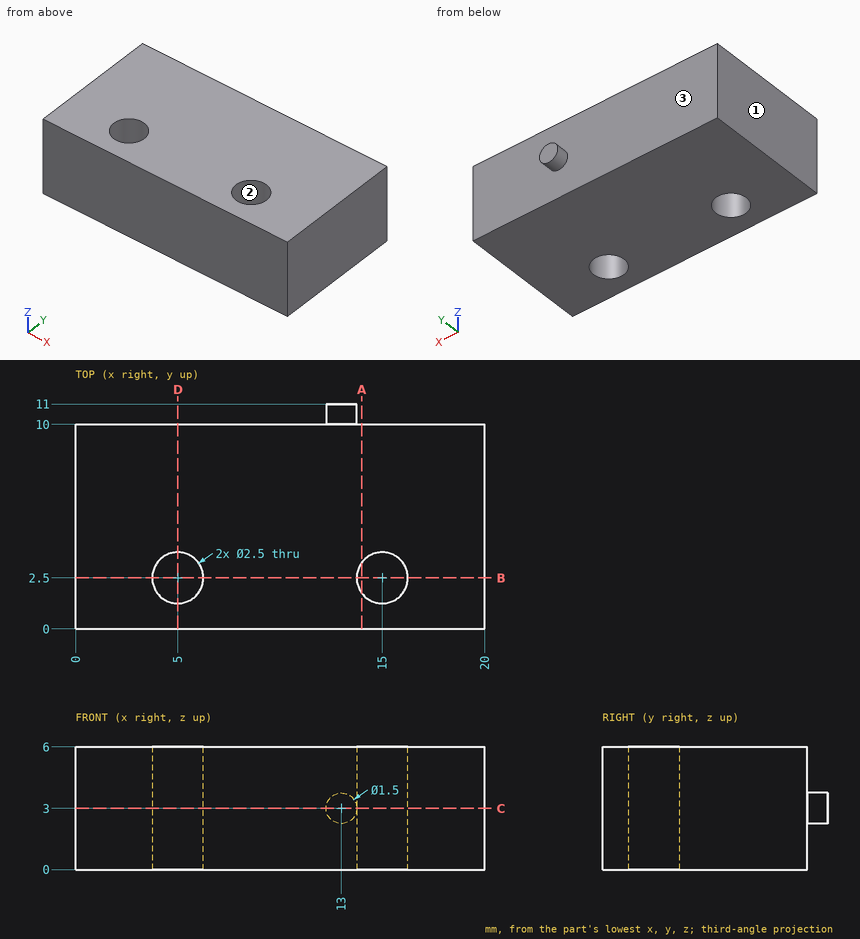
Could you check a few things on this drawing? It's one solid part, dimensions in mm from its lowest x, y, z. Give positions to 0.01 mm unless a question says otherwise; leave off trailing zeros. Write each loop counter-clockwise with the first axis right and the second up, starting at its lowest first coordinate (ties: lowest second). Pieces come first, ordered by that corner, then holes.
(1) Imagine slicing it at C-C, the plane z = 3. Write out the boundary of the cut face in (x, y).
Output values:
outline: (0, 0) - (20, 0) - (20, 10) - (13.75, 10) - (13.75, 11) - (12.25, 11) - (12.25, 10) - (0, 10) - close; hole circle Ø2.5 at (5, 2.5); hole circle Ø2.5 at (15, 2.5)
(2) If I drill on L1, parallel to Y at x = 5, z = 3.4; L2, parallel to X at y = 3.5, z = 4.35; L3, parallel to Y at x = 10.5, z = 1.85, over which ranges is the centre line in solid material (lowest first)?
Output values:
L1: y = 0 to 1.25, 3.75 to 10
L2: x = 0 to 4.25, 5.75 to 14.25, 15.75 to 20
L3: y = 0 to 10
(3) Imagine slicing it at A-A, the plane x = 14. Write out the boundary of the cut face in (y, z), and give its area (3 significant figures).
Output values:
outline: (0, 0) - (1.75, 0) - (1.75, 6) - (0, 6) - close; (3.25, 0) - (10, 0) - (10, 6) - (3.25, 6) - close
area: 51.0 mm2
(4) Will these pins go through, and if not, where does the flat tip stop? pin 1 (2 mm diameter, centred on x = 5, y = 2.5, fed in from -Z); pin 2 (2 mm diameter, centred on x = 15.5, y = 2, fed in from -Z); pin 3 (3 mm diameter, centred on x = 9, z = 4, fed in from +Y).
Output values:
pin 1: passes through
pin 2: stops at z = 0
pin 3: stops at y = 10
(5) Thinking about a two-plate mould opening in Y: for the marked faces 1, 2 and 3, which applies, pulls with the +Y half, pulls with the -Y half, needs draft (parallel to the pull), parting line crosses it, or undercut?
Output values:
face 1: needs draft
face 2: undercut
face 3: pulls with the +Y half
(6) Imagine slicing it at D-D, the plane x = 5. Write out the boundary of the cut face in (y, z), and give its area (3 significant figures).
Output values:
outline: (0, 0) - (1.25, 0) - (1.25, 6) - (0, 6) - close; (3.75, 0) - (10, 0) - (10, 6) - (3.75, 6) - close
area: 45.0 mm2
(7) Imagine slicing it at B-B, the plane y = 2.5. Write out the boundary of the cut face in (x, z).
Output values:
outline: (0, 0) - (3.75, 0) - (3.75, 6) - (0, 6) - close; (6.25, 0) - (13.75, 0) - (13.75, 6) - (6.25, 6) - close; (16.25, 0) - (20, 0) - (20, 6) - (16.25, 6) - close
